The listing builds one solid part. Answer for the finished solid, in the listing's coordinates (mm). Face numbers are marked on the shaded views. A direction names the side the tool comes from. Coordinates: 2 decimals unless noted, no trailing zeros. Order: outer loops, then holes, each group sorted by start corner. A loop starts at its lowest first (then second) coordinate and runs counter-clockwise, first axis right, second up. Notation, with made-up numbers: M 19.5,-25.75 L 66.5,-25.75 A27 ccw 66.5,9.25 Z; hole C 9.25,77 d4. An arc over 180 degrees is marked long. One line per item, written item: value. Start each with the question number.
Q1. For the marked faces 5, 6, 7, 8 and 9, determine the directions among +Z, -Z, +X, -X, +Y, -Y from which every point of the face is accessible in a straight line to the end or side of a thin tool.
Q2. Determine the mould class of the marked faces 1, 2, 3 and 4 for opening direction Z: pulls with the +Z half, pulls with the -Z half, needs draft (parallel to the pull), parting line crosses it, or undercut.
Q3. The part is cut by section D-D on z = 0. Give the vertices of the cut face in (x, y) (3 decimals).
Q4. Each of these flat-tipped pins is pushed along its axis until it touches: pin 1 Ø1.4 at (x, y) = (-2, -2) entering from +Z; pin 2 Ø0.6 at (x, z) = (3.5, 0.5) entering from +Y; pin 3 Ø4 at (x, y) = (-3, -6.5) entering from +Z. Where does it stop, or does it pass through?
Q5. The part is cut by section A-A on z = 6.75. Give the vertices of the cut face in (x, y).
Q6. The part is cut by section B-B on y = -24. Give the vertices of the cut face in (x, z) (3 decimals).
Q7. The part is cut by section C-C on x = 0. Give the vertices of the cut face in (y, z) (3 decimals), then the cut area to 3 significant figures.
Q8. Straight lines are drawn through the part: line 1 along Z through (x, y) = (0, -25) (3 decimals); line 2 along Y through (x, z) = (-6, 2.75). For each, find the intervals that lie inside material, in ascending order. Write a range as [from, to].
Autodesk Inventor part; units mm, degrees
ref_plane "insert_to_lock_XY" through (0, 0, 0) normal (0, 1, 0) x (1, 0, 0)
ref_plane "insert_to_lock_YZ" through (0, 0, 0) normal (1, 0, 0) x (0, 0, -1)
ref_plane "insert_to_lock_ZX" through (0, 0, 0) normal (0, 0, -1) x (0, 1, 0)
sketch "Sketch_1" plane through (0, 0, 0) normal (0, 0, 1) x (1, 0, 0)
  line L0 (0, -20.5) -> (0, 0)
  line L1 (0, 0) -> (7.85, 0)
  line L2 (7.85, 0) -> (7.85, -13.35)
  line L3 (7.85, -13.35) -> (6.375, -13.35)
  line L4 (6.375, -13.35) -> (6.375, -15.85)
  line L5 (6.375, -15.85) -> (7.85, -15.85)
  line L6 (7.85, -15.85) -> (7.85, -17.35)
  line L7 (7.85, -17.35) -> (4.925, -17.35)
  line L8 (4.925, -17.35) -> (4.925, -20.5)
  line L9 (4.925, -20.5) -> (0, -20.5)
  line L10 (0, -20.5) -> (0, 0)
revolve "Revolution1" add sketch "Sketch_1" angle 360 about axis through (0, -20.5, 0) along (0, -1, 0)
sketch "Sketch_2" plane through (0, -20.5, 0) normal (0, 1, 0) x (1, 0, 0)
  arc A0 (-3.4, -2.4) -> (-2.4, -3.4) centre (-2.4, -2.4) ccw
  line L0 (-2.4, -3.4) -> (2.4, -3.4)
  arc A1 (2.4, -3.4) -> (3.4, -2.4) centre (2.4, -2.4) ccw
  line L1 (3.4, -2.4) -> (3.4, 2.4)
  arc A2 (3.4, 2.4) -> (2.4, 3.4) centre (2.4, 2.4) ccw
  line L2 (2.4, 3.4) -> (-2.4, 3.4)
  arc A3 (-2.4, 3.4) -> (-3.4, 2.4) centre (-2.4, 2.4) ccw
  line L3 (-3.4, 2.4) -> (-3.4, -2.4)
  circle A4 centre (0, 0) radius 2.455
extrude "Extrusion1" add sketch "Sketch_2" against normal blind 6.5
sketch "Sketch_3" plane through (0, 0, 0) normal (0, 1, 0) x (-1, 0, 0)
  line L0 (7, -1) -> (7, 1)
  line L1 (7, 1) -> (-7, 1)
  line L2 (-7, 1) -> (-7, -1)
  line L3 (-7, -1) -> (7, -1)
extrude "Extrusion2" cut sketch "Sketch_3" against normal blind 2.71
ref_plane "insert_to_lock_XY" through (0, 0, 0) normal (0, 1, 0) x (1, 0, 0)
ref_plane "insert_to_lock_YZ" through (0, 0, 0) normal (1, 0, 0) x (0, 0, -1)
ref_plane "insert_to_lock_ZX" through (0, 0, 0) normal (0, 0, -1) x (0, 1, 0)
properties part number "lock_insert_na"
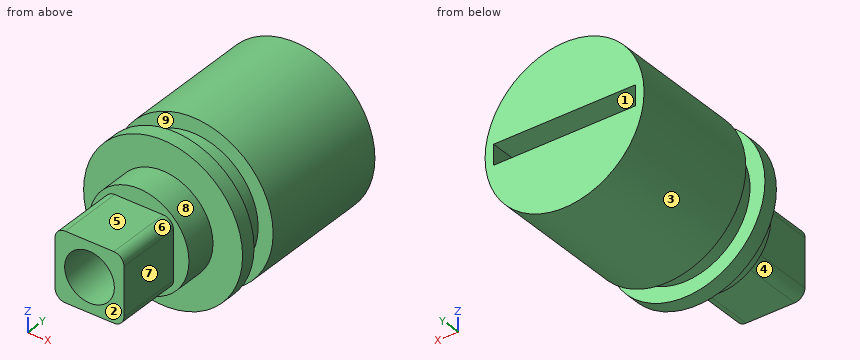
Output:
1. face 5: +Z, +X, -X, -Y
1. face 6: +Z, +X, -Y
1. face 7: +Z, -Z, +X, -Y
1. face 8: -Y
1. face 9: none
2. face 1: undercut
2. face 2: needs draft
2. face 3: parting line crosses it
2. face 4: pulls with the -Z half
3. outline: M -7.85,-17.35 L -4.925,-17.35 L -4.925,-20.5 L -3.4,-20.5 L -3.4,-27 L -2.455,-27 L -2.455,-20.5 L 2.455,-20.5 L 2.455,-27 L 3.4,-27 L 3.4,-20.5 L 4.925,-20.5 L 4.925,-17.35 L 7.85,-17.35 L 7.85,-15.85 L 6.375,-15.85 L 6.375,-13.35 L 7.85,-13.35 L 7.85,0 L 7,0 L 7,-2.71 L -7,-2.71 L -7,0 L -7.85,0 L -7.85,-13.35 L -6.375,-13.35 L -6.375,-15.85 L -7.85,-15.85 Z
4. pin 1: stops at z = 7.74
4. pin 2: stops at y = -2.71
4. pin 3: stops at z = 7.79
5. outline: M -4.01,-17.35 L 4.01,-17.35 L 4.01,-15.85 L -4.01,-15.85 Z; M -4.01,-13.35 L 4.01,-13.35 L 4.01,0 L -4.01,0 Z
6. outline: M -3.4,-2.4 A1 ccw -2.4,-3.4 L 2.4,-3.4 A1 ccw 3.4,-2.4 L 3.4,2.4 A1 ccw 2.4,3.4 L -2.4,3.4 A1 ccw -3.4,2.4 Z; hole C 0,0 d4.91
7. outline: M -27,-3.4 L -20.5,-3.4 L -20.5,-4.925 L -17.35,-4.925 L -17.35,-7.85 L -15.85,-7.85 L -15.85,-6.375 L -13.35,-6.375 L -13.35,-7.85 L 0,-7.85 L 0,-1 L -2.71,-1 L -2.71,1 L 0,1 L 0,7.85 L -13.35,7.85 L -13.35,6.375 L -15.85,6.375 L -15.85,7.85 L -17.35,7.85 L -17.35,4.925 L -20.5,4.925 L -20.5,3.4 L -27,3.4 L -27,2.455 L -20.5,2.455 L -20.5,-2.455 L -27,-2.455 Z
7. area: 303 mm^2
8. line 1: z = [-3.4, -2.455], [2.455, 3.4]
8. line 2: y = [-17.35, -15.85], [-13.35, 0]
